```python
from build123d import *

# Parameters (mm, degrees)
F1_DEPTH = 25.4
F2_R     = 1.5748
F3_DEPTH = 19.05


with BuildPart() as f1:
    # F0 (on Front) → F1 (new body)
    with BuildSketch(Plane.XZ):
        Polygon((-76.2, 0), (0, 0), (-38.1, 65.991136), align=None)
    extrude(amount=F1_DEPTH)

    # F2 (on Front) → F3 (cut)
    with BuildSketch(Plane.XZ):
        with Locations((-38.477365, 54.899465)):
            Circle(F2_R)
        with Locations((-46.49746, 44.01505)):
            Circle(F2_R)
        with Locations((-53.180873, 31.984907)):
            Circle(F2_R)
        with Locations((-61.391924, 17.85426)):
            Circle(F2_R)
        with Locations((-67.502469, 5.442208)):
            Circle(F2_R)
        with Locations((-30.839177, 44.01505)):
            Circle(F2_R)
        with Locations((-38.477365, 31.984907)):
            Circle(F2_R)
        with Locations((-25.301492, 31.984907)):
            Circle(F2_R)
        with Locations((-46.49746, 17.85426)):
            Circle(F2_R)
        with Locations((-30.839177, 17.85426)):
            Circle(F2_R)
        with Locations((-16.517578, 17.85426)):
            Circle(F2_R)
        with Locations((-38.477365, 5.442208)):
            Circle(F2_R)
        with Locations((-53.180873, 5.442208)):
            Circle(F2_R)
        with Locations((-25.301492, 5.442208)):
            Circle(F2_R)
        with Locations((-10.025119, 5.442208)):
            Circle(F2_R)
    extrude(amount=F3_DEPTH, mode=Mode.SUBTRACT)


solid = f1.part
```
Here's how the part is built. I have some questions about the finished solid (model axes, mm). Give positions to 0.01 mm unless a question says otherwise; leave off trailing zeros. Write each loop counter-clockwise with the first axis right and the second up, starting at its lowest first coordinate (ties: lowest second). Pieces come first, ordered by that corner, then holes.
(1) Thinking about a two-plate mould opening in Z: for faces 1 (the face through (-56.88, -12.52, 33.46)), 2 (the face through (-11.186, -9.392, 6.507)), 3 (the face through (-39, -13, 0)), which applies, pulls with the +Z half, pulls with the -Z half, needs draft (parallel to the pull), parting line crosses it, or undercut?
Output values:
face 1: pulls with the +Z half
face 2: undercut
face 3: pulls with the -Z half
(2) Will these pins go through, and if not, where does the flat tip stop? pin 1 (0.9 mm diameter, centred on x = -62, z = 17.5, fed in from +Y); pin 2 (5 mm diameter, centred on y = -6.5, z = 43.5, fed in from +X); pin 3 (1.5 mm diameter, centred on x = -54.5, y = -10.5, fed in from +Z).
Output values:
pin 1: stops at y = -19.05
pin 2: stops at x = -23.67
pin 3: stops at z = 38.88
(3) If I drill on L1, parallel to X at y = -0.75, z = 45; L2, parallel to Z at x = -53.5, y = -16.75; L3, parallel to X at y = -15.25, z = 4.5, over which ranges is the centre line in solid material (lowest first)?
Output values:
L1: x = -50.22 to -47.73, -45.27 to -32.07, -29.61 to -25.98
L2: z = 0 to 3.9, 6.98 to 30.44, 33.53 to 39.32
L3: x = -73.6 to -68.76, -66.24 to -54.44, -51.92 to -39.74, -37.22 to -26.56, -24.04 to -11.29, -8.76 to -2.6
(4) Imagine slicing it at C-C, the plane x = -56. Write out the boundary of the cut face in (y, z), and give its area (3 significant figures).
Output values:
outline: (-25.4, 0) - (0, 0) - (0, 34.99) - (-25.4, 34.99) - close
area: 889 mm2
(5) Imagine slicing it at D-D, the plane z = 59. Write out the boundary of the cut face in (x, y).
Output values:
outline: (-42.14, -25.4) - (-34.06, -25.4) - (-34.06, 0) - (-42.14, 0) - close
(6) Imagine slicing it at A-A, the plane y = -2. Count the separate pieces of the cut face and the enclosed holes in it, and give its area (3 significant figures).
Output values:
separate pieces: 1
enclosed holes: 15
area: 2,400 mm2
(7) Imagine slicing it at B-B, the plane y = -20. Write out the boundary of the cut face in (x, z), and give its area (3 significant figures).
Output values:
outline: (-76.2, 0) - (0, 0) - (-38.1, 65.99) - close
area: 2,510 mm2
